The listing builds one solid part. Answer for the finished solid, in the listing's coordinates (mm). Face numbers are marked on the shaded views. Give positions to 0.01 mm unless a question says otherwise; leave off trailing zeros. Loops run counter-clockwise (first coordinate to the right, second up) from the corner with the lowest first, then second, coordinate; pieces in that order, holes last. Notation, with made-up numbers: (-15.5, 54) - (-2.5, 54) arc R16 cw to (-2.5, 58) - close; hole circle Ø1 at (-24, -27.5). An arc over 180 degrees is marked (long way). Answer in a Markdown table with one row per item. Add a question column.
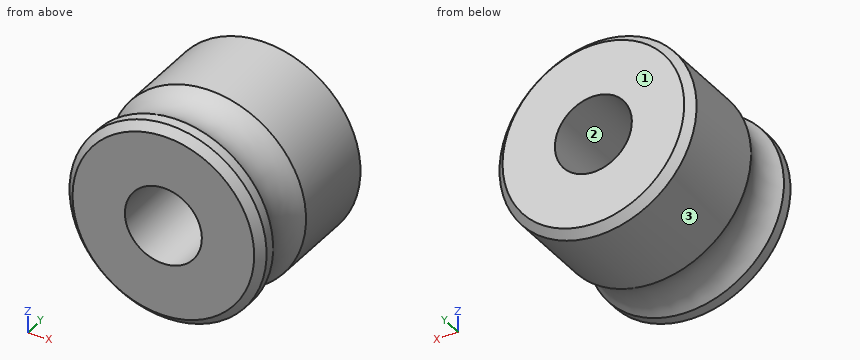
```python
from build123d import *

# Parameters (mm, degrees)
F3_SIZE = 0.5


with BuildPart() as f2:
    # F0 (on Right) → F2 (revolve)
    with BuildSketch(Plane.YZ):
        with BuildLine():
            Line((-5.5, 6.4), (-5.5, 2.5))
            Line((-5.5, 2.5), (5.5, 2.5))
            Line((5.5, 2.5), (5.5, 6.4))
            Line((5.5, 6.4), (-0.8, 6.4))
            ThreePointArc((-0.8, 6.4), (-2.55, 5.836699), (-4.3, 6.4))
            Line((-4.3, 6.4), (-5.5, 6.4))
        make_face()
    revolve(axis=Axis((0, 2.864314, 0), (0, 1, 0)))

    # F3
    f3_edges = [f2.edges().sort_by_distance(p)[0] for p in [
        (0, -5.5, -6.4),
        (0, 5.5, -6.4),
    ]]
    chamfer(f3_edges, length=F3_SIZE)


solid = f2.part
```
(1) A cutting plane is placed at A-A on z = 0. Determine the outline of the cut face in (x, y), plus the area to 3 significant figures.
(2) A cutting plane is placed at B-B on y = 0.25. Determine the outline of the cut face in (x, z), plus the area to 3 significant figures.
(3) A cutting plane is placed at C-C on y = -1.75. Determine the outline of the cut face in (x, z).
(4) The mould has two halves that part along X. Classify the marked faces 1, 2 and 3: pulls with the +X half, pulls with the -X half, needs draft (parallel to the pull), parting line crosses it, or undercut.
(5) Find the intervals of material crossed by line 1 along X through (y, z) = (1.75, 0); line 2 along X through (y, z) = (-4.25, -1); line 3 along Y through (x, z) = (-4.25, 4.25), in increasing order. Write a range as [from, to].
(6) Given pin 1 Ø3 at (x, y) = (3.5, -2) entering from +Z; pin 2 Ø1.5 at (y, z) = (-3.5, -2.5) entering from -X; pin 3 Ø2 at (y, z) = (-3.5, -2.5) entering from -X, each flat-ended and moving along its own axis, determine where each tip first touches the part or whether it passes through.
Evaluation:
| question | item | result |
|---|---|---|
| 1 | outline | (-6.4, -5) - (-5.9, -5.5) - (-2.5, -5.5) - (-2.5, 5.5) - (-5.9, 5.5) - (-6.4, 5) - (-6.4, -0.8) arc R3 cw to (-6.4, -4.3) - close; (2.5, -5.5) - (5.9, -5.5) - (6.4, -5) - (6.4, -4.3) arc R3 cw to (6.4, -0.8) - (6.4, 5) - (5.9, 5.5) - (2.5, 5.5) - close |
| 1 | area | 82.6 mm² |
| 2 | outline | circle Ø12.8 at (0, 0); hole circle Ø5 at (0, 0) |
| 2 | area | 109 mm² |
| 3 | outline | circle Ø11.89 at (0, 0); hole circle Ø5 at (0, 0) |
| 4 | face 1 | needs draft |
| 4 | face 2 | undercut |
| 4 | face 3 | parting line crosses it |
| 5 | line 1 | x = [-6.4, -2.5], [2.5, 6.4] |
| 5 | line 2 | x = [-6.29, -2.29], [2.29, 6.29] |
| 5 | line 3 | y = [-5.39, -3.56], [-1.54, 5.39] |
| 6 | pin 1 | stops at z = 5.85 |
| 6 | pin 2 | stops at x = -5.93 |
| 6 | pin 3 | stops at x = -6.11 |
